Source: CAD feature listing. Evaluate the final solid. Frame: model axes, mm. Give positions to 0.01 mm unless a question says otherwise; leave off trailing zeros. Loops run counter-clockwise (first coordinate to the right, second up) from the corner with the lowest first, then second, coordinate; pieces in that order, holes last. Notation, with made-up numbers: (-24.75, -24.75) -> (29.25, -24.75) arc R17 ccw to (29.25, -6.75) -> close; hole circle Ø8 at (-4, 85). An arc over 180 degrees is marked (long way). Put each result on its own line as item: value.
```python
from build123d import *

# Parameters (mm, degrees)
BOSS_EXTRUDE1_DEPTH   = 470
CHAMFER1_SIZE         = 0.3
LPATTERN1_COUNT       = 12
LPATTERN1_PITCH       = 40
CROQUIS1_W            = 18.891255934
CROQUIS1_H            = 12.405534969
CORTAR_EXTRUIR2_DEPTH = 130
CHAFL_N1_SIZE         = 0.3


with BuildPart() as part:
    # Sketch1 → Boss-Extrude1 (new body)
    with BuildSketch(Plane.XY):
        with BuildLine():
            Line((0, 8), (12, 8))
            Line((12, 8), (12, 6.75))
            Line((12, 6.75), (12, 6.559016994))
            ThreePointArc((12, 6.559016994), (11.706107374, 6.475528258), (11.5, 6.25))
            Line((11.5, 6.25), (11, 6.25))
            Line((11, 6.25), (11, 5.75))
            Line((11, 5.75), (11.5, 5.75))
            ThreePointArc((11.5, 5.75), (11.706107374, 5.524471742), (12, 5.440983006))
            Line((12, 5.440983006), (12, 5.25))
            Line((12, 5.25), (12, 0))
            Line((12, 0), (0, 0))
            Line((0, 0), (0, 5.25))
            Line((0, 5.25), (0, 5.440983006))
            ThreePointArc((0, 5.440983006), (0.293892626, 5.524471742), (0.5, 5.75))
            Line((0.5, 5.75), (1, 5.75))
            Line((1, 5.75), (1, 6.25))
            Line((1, 6.25), (0.5, 6.25))
            ThreePointArc((0.5, 6.25), (0.293892626, 6.475528258), (0, 6.559016994))
            Line((0, 6.559016994), (0, 6.75))
            Line((0, 6.75), (0, 8))
        make_face()
    extrude(amount=BOSS_EXTRUDE1_DEPTH)

    # Chamfer1
    chamfer1_edges = [part.edges().sort_by_distance(p)[0] for p in [
        (12, 2.720491503, 470),
        (11.706107374, 5.524471742, 470),
        (0, 2.720491503, 0),
        (0.293892626, 5.524471742, 0),
        (0.75, 5.75, 0),
        (1, 6, 0),
        (0.75, 6.25, 0),
        (11.25, 5.75, 470),
        (0.293892626, 6.475528258, 0),
        (0, 7.279508497, 0),
        (6, 8, 0),
        (12, 7.279508497, 0),
        (11.706107374, 6.475528258, 0),
        (11, 6, 470),
        (11.25, 6.25, 0),
        (11, 6, 0),
        (11.25, 5.75, 0),
        (11.706107374, 5.524471742, 0),
        (12, 2.720491503, 0),
        (6, 0, 0),
        (11.25, 6.25, 470),
        (11.706107374, 6.475528258, 470),
        (12, 7.279508497, 470),
        (0, 8, 235),
        (12, 8, 235),
        (12, 0, 235),
        (0, 0, 235),
        (6, 8, 470),
        (0, 2.720491503, 470),
        (0, 7.279508497, 470),
        (0.293892626, 6.475528258, 470),
        (0.75, 6.25, 470),
        (1, 6, 470),
        (0.75, 5.75, 470),
        (0.293892626, 5.524471742, 470),
        (6, 0, 470),
    ]]
    chamfer(chamfer1_edges, length=CHAMFER1_SIZE)

    # Sketch3 → CBORE for M5 Hex Head Bolt1 (revolve, cut)
    with BuildSketch(Plane(origin=(6, 8, 15), x_dir=(0, 0, 1), z_dir=(1, 0, 0))):
        Polygon((0, 0), (0, 8), (2.5, 8), (2.25, 7.75), (2.25, 4.5), (4, 4.5), (4, 0.25), (4.25, 0), align=None)
    cbore_for_m5_hex_head_bolt1 = revolve(axis=Axis((6, 14.35, 15), (0, -1, 0)), mode=Mode.SUBTRACT)

    # LPattern1: CBORE for M5 Hex Head Bolt1 ×12
    with Locations(*[(0, 0, i * LPATTERN1_PITCH) for i in range(1, LPATTERN1_COUNT)]):
        add(cbore_for_m5_hex_head_bolt1, mode=Mode.SUBTRACT)

    # Croquis1 → Cortar-Extruir2 (cut)
    with BuildSketch(Plane.XY.offset(470)):
        with Locations((5.286012754, 3.624640076)):
            Rectangle(CROQUIS1_W, CROQUIS1_H)
    extrude(amount=-CORTAR_EXTRUIR2_DEPTH, mode=Mode.SUBTRACT)

    # Chaflán1
    chafl_n1_edges = [part.edges().sort_by_distance(p)[0] for p in [
        (0.15, 0.15, 340),
        (11.85, 0.15, 340),
        (0.15, 7.85, 340),
        (11.85, 7.85, 340),
        (12, 2.870491503, 340),
        (11.706107374, 5.524471742, 340),
        (11.25, 5.75, 340),
        (11, 6, 340),
        (11.25, 6.25, 340),
        (11.706107374, 6.475528258, 340),
        (12, 7.129508497, 340),
        (6, 8, 340),
        (0, 7.129508497, 340),
        (0.293892626, 6.475528258, 340),
        (0.75, 6.25, 340),
        (1, 6, 340),
        (0.75, 5.75, 340),
        (0.293892626, 5.524471742, 340),
        (0, 2.870491503, 340),
        (6, 0, 340),
    ]]
    chamfer(chafl_n1_edges, length=CHAFL_N1_SIZE)


solid = part.part
```
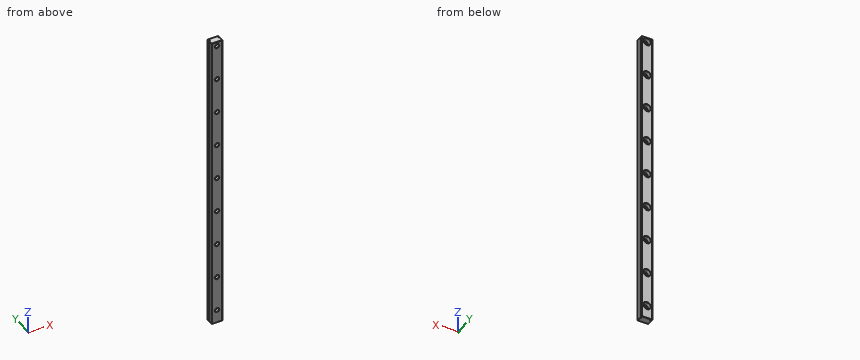
(1) First-contact query: P1, Ø6.5, axis at x = 6, z = 335, coming from the +Y side. Flat tip, straight axial feed; report the tip coordinate or a pass-through.
Calculated:
P1: stops at y = 3.5
(2) Section B-B on z = 163. Return loops of the section in (x, y), then the cut area to 3 significant figures.
Calculated:
outline: (0, 0.3) -> (0.3, 0) -> (11.7, 0) -> (12, 0.3) -> (12, 5.44) arc R0.56 cw to (11.5, 5.75) -> (11, 5.75) -> (11, 6.25) -> (11.5, 6.25) arc R0.56 cw to (12, 6.56) -> (12, 7.7) -> (11.7, 8) -> (0.3, 8) -> (0, 7.7) -> (0, 6.56) arc R0.56 cw to (0.5, 6.25) -> (1, 6.25) -> (1, 5.75) -> (0.5, 5.75) arc R0.56 cw to (0, 5.44) -> close
area: 94.4 mm²
(3) Line query: probe 1 along Y at (x, z) = (0.75, 81.5); probe 2 along X at (y, z) = (4.9, 335); probe 3 along Y at (x, z) = (11.75, 272). Output: solid intervals per line, ascending. Write a range as from..to.
Calculated:
probe 1: y = 0..5.75, 6.25..8
probe 2: x = 0..2, 10..12
probe 3: y = 0.05..5.5, 6.5..7.95
(4) Section A-A on y = 2. Give the number of separate pieces and of enclosed holes in the cut face, then the cut area to 3 significant figures.
Calculated:
separate pieces: 1
enclosed holes: 9
area: 3,940 mm²
